from build123d import *

# Parameters (mm, degrees)
SKETCH1_W           = 28
SKETCH1_H           = 28
BOSS_EXTRUDE1_DEPTH = 33
SKETCH3_W           = 49.200789626
SKETCH3_H           = 42.103599699
CUT_EXTRUDE1_DEPTH  = 15
FILLET1_R           = 2
SKETCH7_W           = 35.932527634
SKETCH7_H           = 14.196879105
CUT_EXTRUDE3_DEPTH  = 2
SHELL1_START        = -12
SHELL1_DEPTH        = 26
SKETCH8_R           = 1.7
CUT_EXTRUDE4_DEPTH  = 2
SKETCH9_R           = 1.590347025
SKETCH9_R_2         = 1.7
CUT_EXTRUDE5_DEPTH  = 2


# Read off the part's stored shape, not the designer's step: Shell1
with BuildPart() as part:
    # Sketch1 → Boss-Extrude1 (new body)
    with BuildSketch(Plane.XY):
        Rectangle(SKETCH1_W, SKETCH1_H)
    extrude(amount=BOSS_EXTRUDE1_DEPTH)

    # Sketch3 → Cut-Extrude1 (cut)
    with BuildSketch(Plane(origin=(2.500486732, 0, 5.362311102), x_dir=(0, 1, 0), z_dir=(0.4226182617407003, 0, 0.9063077870366496))):
        with Locations((-1.181385954, 1.948035585)):
            Rectangle(SKETCH3_W, SKETCH3_H)
    extrude(amount=-CUT_EXTRUDE1_DEPTH, mode=Mode.SUBTRACT)

    # Fillet1
    fillet1_edges = [part.edges().sort_by_distance(p)[0] for p in [
        (14, -14, 16.5),
        (-14, -14, 23.028307214),
        (-14, 14, 23.028307214),
        (14, 14, 16.5),
    ]]
    fillet(fillet1_edges, radius=FILLET1_R)

    # Sketch7 → Cut-Extrude3 (cut)
    with BuildSketch(Plane(origin=(11.499513268, 0, -5.362311102), x_dir=(0, 1, 0), z_dir=(0.9063077870366496, 0, -0.4226182617407003))):
        with Locations((0.607628843, 7.098439553)):
            Rectangle(SKETCH7_W, SKETCH7_H)
    extrude(amount=-CUT_EXTRUDE3_DEPTH, mode=Mode.SUBTRACT)

    # Shell1 outline → Shell1 (cut)
    with BuildSketch(Plane(origin=(0, 0, 0), x_dir=(1, 0, 0), z_dir=(0, 1, 0)).offset(SHELL1_START)):
        Polygon((12, -31), (12, -5.175792492), (11.220005375, -3.503088621), (-12, -14.33075495), (-12, -31), align=None)
    extrude(amount=SHELL1_DEPTH, mode=Mode.SUBTRACT)

    # Sketch8 → Cut-Extrude4 (cut)
    with BuildSketch(Plane.XY.offset(33)):
        with Locations((-8, 8)):
            Circle(SKETCH8_R)
        with Locations((8, 8)):
            Circle(SKETCH8_R)
        with Locations((8, -8)):
            Circle(SKETCH8_R)
        with Locations((-8, -8)):
            Circle(SKETCH8_R)
    extrude(amount=-CUT_EXTRUDE4_DEPTH, mode=Mode.SUBTRACT)

    # Sketch9 → Cut-Extrude5 (cut)
    with BuildSketch(Plane(origin=(2.500486732, 0, 5.362311102), x_dir=(-0.9063077870366496, 0, 0.4226182617407002), z_dir=(-0.4226182617407003, 0, -0.9063077870366497))):
        with Locations((11.206272712, -8)):
            Circle(SKETCH9_R)
        with Locations((11.206272712, 8)):
            Circle(SKETCH9_R_2)
        with Locations((-6.293727288, 0)):
            Circle(SKETCH9_R_2)
    extrude(amount=-CUT_EXTRUDE5_DEPTH, mode=Mode.SUBTRACT)


solid = part.part
Source: CAD feature listing. Evaluate the final solid. Frame: model axes, mm. A direction names the side the tool comes from. Coordinates: 2 decimals unless noted, no trailing zeros. Loops run counter-clockwise (first coordinate to the right, second up) from the corner with the lowest first, then second, coordinate; pieces in that order, holes last. Notation, with made-up numbers: M -37.75,85.25 L 2.25,85.25 A22 ccw 2.25,113.25 Z; hole C -30.75,-14 d5. An arc over 180 degrees is marked long. Answer in a Markdown table with one row per item.
Q1. Section D-D on y = -8. Return the cut outline in (x, z).
Answers below:
| item | result |
|---|---|
| outline | M -14,13.06 L -9.1,10.77 L -8.25,12.58 L -12,14.33 L -12,31 L -9.7,31 L -9.7,33 L -14,33 Z; M -6.3,31 L 6.3,31 L 6.3,33 L -6.3,33 Z; M -6.21,9.43 L 12.19,0.85 L 14,4.73 L 14,33 L 9.7,33 L 9.7,31 L 12,31 L 12,5.18 L 11.22,3.5 L -5.37,11.24 Z |
Q2. Section B-B on y = 8. Return the cut outline in (x, z), plus the area to 3 significant figures.
Answers below:
| item | result |
|---|---|
| outline | M -14,13.06 L -9.2,10.82 L -8.35,12.63 L -12,14.33 L -12,31 L -9.7,31 L -9.7,33 L -14,33 Z; M -6.3,31 L 6.3,31 L 6.3,33 L -6.3,33 Z; M -6.12,9.38 L 12.19,0.85 L 14,4.73 L 14,33 L 9.7,33 L 9.7,31 L 12,31 L 12,5.18 L 11.22,3.5 L -5.27,11.19 Z |
| area | 183 mm^2 |
Q3. Ray query, probe 1 along Y at (x, z) = (8, 31.5); probe 2 along X at (y, z) = (12.25, 16); probe 3 along Y at (x, z) = (0, 21.5). Return the intervals inside material, ascending. Write a range as from..to.
Answers below:
| item | result |
|---|---|
| probe 1 | y = -14..-9.7, -6.3..6.3, 9.7..14 |
| probe 2 | x = -13.98..-12, 12..13.98 |
| probe 3 | y = -14..-12 |
Q4. First-contact query: pin 1 (5.5 mm diameter, centred on x = 8, y = 8, fed in from -Z); pin 2 (2.5 mm diameter, centred on x = -8, y = 8, fed in from +Z); pin 3 (10 mm diameter, centred on x = -6, y = 10, fed in from -Z). Flat tips, straight axial feed; report the tip coordinate or a pass-through.
Answers below:
| item | result |
|---|---|
| pin 1 | stops at z = 1.52 |
| pin 2 | stops at z = 13.05 |
| pin 3 | stops at z = 6.99 |
Q5. Section A-A on z = 26. Return the cut outline in (x, y).
Answers below:
| item | result |
|---|---|
| outline | M -14,-12 A2 ccw -12,-14 L 12,-14 A2 ccw 14,-12 L 14,12 A2 ccw 12,14 L 12,-12 L -12,-12 L -12,14 A2 ccw -14,12 Z |
Q6. Set-up query: faces 4 (the cylindrical face through (-8.37, -9.66, 32.01)), 5 (the cylindrical face through (-13.43, 13.4, 22.71)), 6 (the flat face through (12, 1, 18)). Return all of +Z, -Z, +X, -X, +Y, -Y with unobstructed straight access to the full face (end or side cutting, diameter ignored); none if empty.
Answers below:
| item | result |
|---|---|
| face 4 | +Z |
| face 5 | +Z, -Z, -X, +Y |
| face 6 | +Y |
Q7. Draft query along X for faces 1 (the flat face through (0, 1, 31)), 2 (the cylindrical face through (13.4, -13.43, 17.15)), 3 (the flat face through (0, -14, 20)). Return one class per face: pulls with the +X half, pulls with the -X half, needs draft (parallel to the pull), parting line crosses it, or undercut.
Answers below:
| item | result |
|---|---|
| face 1 | undercut |
| face 2 | pulls with the +X half |
| face 3 | needs draft |
Q8. Section C-C on x = -10.5. Return the cut outline in (y, z).
Answers below:
| item | result |
|---|---|
| outline | M -14,11.42 L 14,11.42 L 14,13.63 L -12,13.63 L -12,31 L 14,31 L 14,33 L -14,33 Z |
